from build123d import *

# Parameters (mm, degrees)
F0_W      = 268.8
F0_H      = 218
F4_DEPTH  = 711.2
F5_DEPTH  = 406.4
F2_W      = 268.8
F2_H      = 268.8
F6_DEPTH  = 304.8
F3_W      = 18
F3_H      = 1016
F7_DEPTH  = 406.4
F9_DEPTH  = 25.4
F10_DEPTH = 330.201
F11_W     = 304.8
F11_H     = 1828.8
F12_DEPTH = 9


with BuildPart() as f4:
    # F0 (on Front) → F4 (new body)
    with BuildSketch(Plane.XZ):
        Polygon((0, 254), (0, 0), (304.8, 0), (304.8, 254), (286.8, 254), (18, 254), align=None)
        with Locations((152.4, 127)):
            Rectangle(F0_W, F0_H, mode=Mode.SUBTRACT)
    extrude(amount=F4_DEPTH)

    # F1 (on face) → F5 (join)
    with BuildSketch(Plane.XZ):
        Polygon((0, 254), (18, 254), (18, 490), (286.8, 490), (286.8, 254), (304.8, 254), (304.8, 508), (0, 508), align=None)
    extrude(amount=F5_DEPTH)



with BuildPart() as f6:
    # F2 (on face) → F6 (new body)
    with BuildSketch(Plane.XZ):
        Polygon((286.8, 1524), (304.8, 1524), (304.8, 1828.8), (0, 1828.8), (0, 1524), (18, 1524), align=None)
        with Locations((152.4, 1676.4)):
            Rectangle(F2_W, F2_H, mode=Mode.SUBTRACT)
    extrude(amount=F6_DEPTH)


with BuildPart() as f4_1:
    add(f4.part)

    add(f6.part)  # F7 merges F6
    # F3 (on face) → F7 (join)
    with BuildSketch(Plane.XZ):
        with Locations((9, 1016)):
            Rectangle(F3_W, F3_H)
        with Locations((295.8, 1016)):
            Rectangle(F3_W, F3_H)
    extrude(amount=F7_DEPTH)

    # F8 (on face) → F9 (join)
    with BuildSketch(Plane.YZ.offset(304.8)):
        with BuildLine():
            Line((-406.4, 1524), (-406.4, 508))
            add(Edge.make_bspline(
                [(-406.4, 508), (-396.8275922681, 598.5997341904), (-421.7207556926, 754.4937009727), (-111.9974998318, 1301.6475166208), (-304.8, 1524)],
                knots=[0, 0, 0, 0, 0.3701888658, 1, 1, 1, 1], degree=3))
            Line((-304.8, 1524), (-406.4, 1524))
        make_face()
    extrude(amount=F9_DEPTH)

    # F10 (cut, through all): a face of the model
    f10_faces = [f4_1.faces().sort_by_distance(p)[0] for p in [
        (330.2, -333.081689218, 1181.2920235829),
    ]]
    extrude(f10_faces, amount=-F10_DEPTH, mode=Mode.SUBTRACT)

    # F11 (on face) → F12 (join)
    with BuildSketch(Plane(origin=(0, 0, 0), x_dir=(-1, 0, 0), z_dir=(0, 1, 0))):
        with Locations((-152.4, 914.4)):
            Rectangle(F11_W, F11_H)
    extrude(amount=F12_DEPTH)


solid = f4_1.part
The listing builds one solid part. Answer for the finished solid, in the listing's coordinates (mm). A direction names the side the tool comes from. Coordinates: 2 decimals unless noted, no trailing zeros. Order: outer loops, then holes, each group sorted by start corner. A loop starts at its lowest first (then second) coordinate and runs counter-clockwise, first axis right, second up.
Q1. A cutting plane is placed at D-D, the plane y = -486.5. Write down the section's boundary in (x, z).
Q2. Consider line 1 (Z direction, x = 174, y = -177); line 2 (Z direction, x = 73, y = -406); line 3 (X direction, y = -474, z = 152). Determine where each line is inside the solid, lowest interval first.
Q3. A cutting plane is placed at A-A, the plane x = 197.5. Write down the section's boundary in (y, z), and give its area (3 significant figures).
Q4. A cutting plane is placed at B-B, the plane z = 1677. Write down the section's boundary in (x, y), and give its area (3 significant figures).
Q5. Which of the six approach directions +Z, -Z, +X, -X, +Y, -Y give full straight-line access (tool end or side, diameter ignored) to faces 4 (the face through (155, 9, 927)), 5 (the face through (18, -200, 370)), 6 (the face through (163, -406.4, 494))?
Q6. Given P1, Ø2, axis at x = 52.5, y = -516, coming from the +Z side, flat-ended and moving along its own axis, determine where the tip first touches the part or whether it passes through.
Q7. For a pull along X with two mould halves and no side action, classify faces 1 (the face through (151, -150, 1810.8)), 2 (the face through (16, -304.8, 1677)), 3 (the face through (304.8, -196, 698)) as pulls with the +X half, pulls with the -X half, needs draft (parallel to the pull), parting line crosses it, or undercut.
Q8. A cutting plane is placed at C-C, the plane y = -49. Write down the section's boundary in (x, z), and give its area (3 significant figures).
Answers follow:
1. outline: (0, 0) - (304.8, 0) - (304.8, 254) - (0, 254) - close; hole (18, 18) - (286.8, 18) - (286.8, 236) - (18, 236) - close
2. line 1: z = 0 to 18, 236 to 254, 490 to 508, 1524 to 1542, 1810.8 to 1828.8
2. line 2: z = 0 to 18, 236 to 254, 490 to 508
2. line 3: x = 0 to 18, 286.8 to 304.8
3. outline: (-711.2, 0) - (9, 0) - (9, 1828.8) - (-304.8, 1828.8) - (-304.8, 1810.8) - (0, 1810.8) - (0, 1542) - (-304.8, 1542) - (-304.8, 1524) - (0, 1524) - (0, 508) - (-406.4, 508) - (-406.4, 490) - (0, 490) - (0, 254) - (-711.2, 254) - (-711.2, 236) - (0, 236) - (0, 18) - (-711.2, 18) - close
3. area: 60,400 mm2
4. outline: (0, -304.8) - (18, -304.8) - (18, 0) - (286.8, 0) - (286.8, -304.8) - (304.8, -304.8) - (304.8, 9) - (0, 9) - close
4. area: 13,700 mm2
5. face 4: +Z, -Z, +X, -X, +Y
5. face 5: -Y
5. face 6: +Z, +X, -X, -Y
6. P1: stops at z = 254
7. face 1: undercut
7. face 2: needs draft
7. face 3: pulls with the +X half
8. outline: (0, 0) - (304.8, 0) - (304.8, 1828.8) - (0, 1828.8) - close; hole (18, 18) - (286.8, 18) - (286.8, 236) - (18, 236) - close; hole (18, 254) - (286.8, 254) - (286.8, 490) - (18, 490) - close; hole (18, 508) - (286.8, 508) - (286.8, 1524) - (18, 1524) - close; hole (18, 1542) - (286.8, 1542) - (286.8, 1810.8) - (18, 1810.8) - close
8. area: 90,000 mm2
